Read the model definition and answer for the solid it produces. Units are mm, in the model's axes. Face numbers are marked on the shaded views. A direction names the side the tool comes from. Coordinates: 2 decimals unless noted, no trailing zeros. Loops run counter-clockwise (first coordinate to the right, second up) from the corner with the lowest first, then second, coordinate; pieces in that order, holes last. Notation, with made-up numbers: (70, 21) -> (104, 21) arc R14 ccw to (104, 28) -> close; hole circle Ø3 at (57, -38). An arc over 180 degrees is marked (long way). Answer as CSV lines item,"result".
```python
from build123d import *

# Parameters (mm, degrees)
CROQUIS2_W              = 65
CROQUIS2_H              = 35
CROQUIS2_W_2            = 35
CROQUIS2_H_2            = 25
SALIENTE_EXTRUIR1_DEPTH = 20
CROQUIS3_R              = 12.5
CORTAR_EXTRUIR1_DEPTH   = 60
CROQUIS4_R              = 6.5
CORTAR_EXTRUIR2_DEPTH   = 5
CROQUIS10_R             = 50
CROQUIS10_R_2           = 44.640302452
SALIENTE_EXTRUIR2_DEPTH = 20
CROQUIS11_W             = 65
CROQUIS11_H             = 10
CROQUIS11_R             = 1.5
SALIENTE_EXTRUIR3_DEPTH = 10
SALIENTE_EXTRUIR4_DEPTH = 2.5


with BuildPart() as part:
    # Croquis2 → Saliente-Extruir1 (new body)
    with BuildSketch(Plane(origin=(0, 0, 0), x_dir=(1, 0, 0), z_dir=(0, 1, 0))):
        with Locations((17.5, 12.5)):
            Rectangle(CROQUIS2_W, CROQUIS2_H)
        with Locations((17.5, 12.5)):
            Rectangle(CROQUIS2_W_2, CROQUIS2_H_2, mode=Mode.SUBTRACT)
    extrude(amount=SALIENTE_EXTRUIR1_DEPTH)

    # Croquis3 → Cortar-Extruir1 (cut)
    with BuildSketch(Plane(origin=(50, 0, 0), x_dir=(0, 0, -1), z_dir=(1, 0, 0))):
        with Locations((12.5, 0)):
            Circle(CROQUIS3_R)
    extrude(amount=-CORTAR_EXTRUIR1_DEPTH, mode=Mode.SUBTRACT)

    # Croquis4 → Cortar-Extruir2 (cut)
    with BuildSketch(Plane.ZY.offset(15)):
        with Locations((-12.5, 0)):
            Circle(CROQUIS4_R)
    extrude(amount=-CORTAR_EXTRUIR2_DEPTH, mode=Mode.SUBTRACT)

    # Croquis5 → Recubrir2 section 0
    with BuildSketch(Plane(origin=(0, 20, 0), x_dir=(1, 0, 0), z_dir=(0, 1, 0))):
        with BuildLine():
            Line((-15, -5), (50, -5))
            Line((50, -5), (50, 30))
            Line((50, 30), (-15, 30))
            Line((-15, 30), (-15, -5))
        make_face()
    # Croquis6 for Recubrir2 → Recubrir2 section 1
    with BuildSketch(Plane(origin=(0, 60, 0), x_dir=(1, 0, 0), z_dir=(0, 1, 0))):
        with BuildLine():
            # circular arc as an exact rational Bezier (weights 1, cos(half-angle), 1)
            Bezier((-26.523554996, -11.204991152), (17.5, -92.963021858), (61.523554996, -11.204991152), weights=[1, 0.474099823, 1])
            Bezier((61.523554996, -11.204991152), (74.287781001, 12.5), (61.523554996, 36.204991152), weights=[1, 0.8804711, 1])
            Bezier((61.523554996, 36.204991152), (17.5, 117.963021858), (-26.523554996, 36.204991152), weights=[1, 0.474099823, 1])
            Bezier((-26.523554996, 36.204991152), (-39.287781001, 12.5), (-26.523554996, -11.204991152), weights=[1, 0.8804711, 1])
        make_face()
    loft()

    # Croquis10 → Saliente-Extruir2 (add)
    with BuildSketch(Plane(origin=(0, 60, 0), x_dir=(1, 0, 0), z_dir=(0, 1, 0))):
        with Locations(Location((17.5, 12.5, 0), (0, 0, 151.699244219))):
            Circle(CROQUIS10_R)
        with Locations(Location((17.5, 12.5, 0), (0, 0, 270))):
            Circle(CROQUIS10_R_2, mode=Mode.SUBTRACT)
    extrude(amount=SALIENTE_EXTRUIR2_DEPTH)

    # Croquis11 → Saliente-Extruir3 (add)
    # profile 1 of 2: a face of its own
    with BuildSketch(Plane.XZ):
        with Locations((17.5, 10)):
            Rectangle(CROQUIS11_W, CROQUIS11_H)
        with Locations(Location((45, 10, 0), (0, 0, 270))):
            Circle(CROQUIS11_R, mode=Mode.SUBTRACT)
        with Locations(Location((-10, 10, 0), (0, 0, 270))):
            Circle(CROQUIS11_R, mode=Mode.SUBTRACT)
        with Locations(Location((17.5, 10, 0), (0, 0, 270))):
            Circle(CROQUIS11_R, mode=Mode.SUBTRACT)
    # profile 2 of 2: a face of its own
    with BuildSketch(Plane.XZ):
        with Locations((17.5, -35)):
            Rectangle(CROQUIS11_W, CROQUIS11_H)
        with Locations(Location((45, -35, 0), (0, 0, 270))):
            Circle(CROQUIS11_R, mode=Mode.SUBTRACT)
        with Locations(Location((-10, -35, 0), (0, 0, 270))):
            Circle(CROQUIS11_R, mode=Mode.SUBTRACT)
        with Locations(Location((17.5, -35, 0), (0, 0, 270))):
            Circle(CROQUIS11_R, mode=Mode.SUBTRACT)
    extrude(amount=-SALIENTE_EXTRUIR3_DEPTH)

    # Croquis12 → Saliente-Extruir4 (add, symmetric)
    with BuildSketch(Plane(origin=(31.25, 0, 0), x_dir=(0, 0, -1), z_dir=(1, 0, 0))):
        Polygon((-5, 10), (-5, 50), (-25, 50), (-15, 10), align=None)
        Polygon((30, 10), (40, 10), (50.3125, 50), (30, 50), align=None)
    saliente_extruir4 = extrude(amount=SALIENTE_EXTRUIR4_DEPTH, both=True)

    # Simetría1: Saliente-Extruir4 across plane
    add(saliente_extruir4.mirror(Plane(origin=(17.5, 0, 0), x_dir=(0, 0, 1), z_dir=(1, 0, 0))))

    # Croquis9 → Cortar-Recubrir2 section 0
    with BuildSketch(Plane(origin=(0, 20, 0), x_dir=(1, 0, 0), z_dir=(0, 1, 0))):
        with BuildLine():
            Line((0, 0), (35, 0))
            Line((35, 0), (35, 25))
            Line((35, 25), (0, 25))
            Line((0, 25), (0, 0))
        make_face()
    # Croquis8 for Cortar-Recub → Cortar-Recubrir2 section 1
    with BuildSketch(Plane(origin=(0, 60, 0), x_dir=(1, 0, 0), z_dir=(0, 1, 0))):
        with BuildLine():
            Bezier((-18.82530827, -13.446648764), (17.5, -64.302080343), (53.82530827, -13.446648764), weights=[1, 0.581238194, 1])
            Bezier((53.82530827, -13.446648764), (72.358628816, 12.5), (53.82530827, 38.446648764), weights=[1, 0.813733471, 1])
            Bezier((53.82530827, 38.446648764), (17.5, 89.302080343), (-18.82530827, 38.446648764), weights=[1, 0.581238194, 1])
            Bezier((-18.82530827, 38.446648764), (-37.358628816, 12.5), (-18.82530827, -13.446648764), weights=[1, 0.813733471, 1])
        make_face()
    loft(mode=Mode.SUBTRACT)


solid = part.part
```
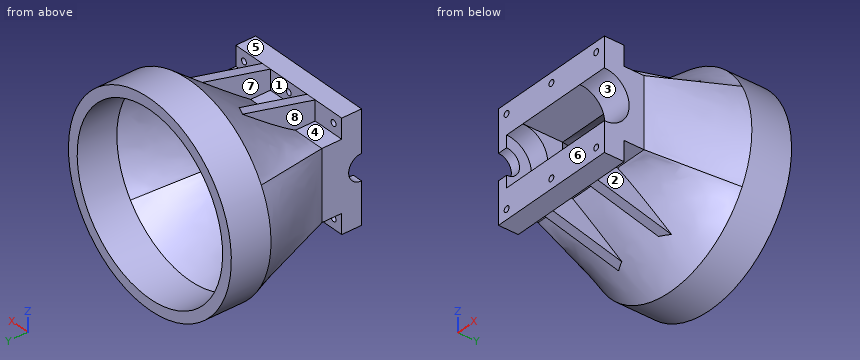
Q1. For a pull along X with two mould halves and no side action, classify the marked faces 6, 7 and 8 as pulls with the +X half, pulls with the -X half, needs draft (parallel to the pull), parting line crosses it, or undercut.
Results:
face 6,"needs draft"
face 7,"undercut"
face 8,"pulls with the -X half"
Q2. Given pin 1 Ø1.5 at (y, z) = (49, -20.5) entering from +X; pin 2 Ø12 at (x, y) = (-13.5, 41) entering from -Z; pin 3 Ø4 at (y, z) = (11.5, 9) entering from -X, each flat-ended and moving along its own axis, determine where each tip first touches the part or whether it passes through.
Results:
pin 1,"stops at x = 62.47"
pin 2,"stops at z = -43.63"
pin 3,"stops at x = -15"
Q3. A cutting plane is placed at D-D, the plane y = 74.5. Write down the section's boundary in (x, z) (3 decimals).
Results:
outline,"circle Ø100 at (17.5, -12.5); hole circle Ø89.281 at (17.5, -12.5)"
Q4. Find the intervals of material crossed by probe 1 along X at (y, z) = (7.5, -35); probe 2 along Z at (x, y) = (6.5, 7.5); probe 3 along Z at (x, y) = (27, 13.5), in increasing order. Write a range as [from, to].
Results:
probe 1,"x = [-15, -11.5], [-8.5, 16], [19, 43.5], [46.5, 50]"
probe 2,"z = [-40, -25], [0, 15]"
probe 3,"z = [-30, -25], [0, 5]"
Q5. For the marked faces 1, 2, 3, 4 and 5, determine the directions among +Z, -Z, +X, -X, +Y, -Y from which every point of the face is accessible in a straight line to the end or side of a thin tool.
Results:
face 1,"+Z"
face 2,"-Z, +X"
face 3,"+X, -Y"
face 4,"+Z, -X"
face 5,"+Z, +X, -X, -Y"
Q6. A cutting plane is placed at B-B, the plane y = 15.5. Write down the section's boundary in (x, z) (3 decimals), and give its area (3 significant figures).
Results:
outline,"(-15, -30) -> (1.25, -30) -> (1.25, -41.418) -> (6.25, -41.418) -> (6.25, -30) -> (28.75, -30) -> (28.75, -41.418) -> (33.75, -41.418) -> (33.75, -30) -> (50, -30) -> (50, 5) -> (33.75, 5) -> (33.75, 16.375) -> (28.75, 16.375) -> (28.75, 5) -> (6.25, 5) -> (6.25, 16.375) -> (1.25, 16.375) -> (1.25, 5) -> (-15, 5) -> close; hole (0, -25) -> (35, -25) -> (35, 0) -> (0, 0) -> close"
area,"1,630 mm²"
Q7. A cutting plane is placed at A-A, the plane x = 17.5. Give the number of separate pieces and of enclosed holes in the cut face, and give its area (3 significant figures).
Results:
separate pieces,"4"
enclosed holes,"0"
area,"969 mm²"
